Autodesk Inventor part; units mm, degrees
ref_plane "YZ Plane" through (0, 0, 0) normal (1, 0, 0) x (0, 1, 0)
ref_plane "XZ Plane" through (0, 0, 0) normal (0, 1, 0) x (-1, 0, 0)
ref_plane "XY Plane" through (0, 0, 0) normal (0, 0, 1) x (1, 0, 0)
sketch "Boceto2" plane through (0, 0, 0) normal (0, 0, 1) x (1, 0, 0)
  circle A0 centre (0, 0) radius 7.9375
  dimension "d0" = 15.875
extrude "Extrusión1" add sketch "Boceto2" against normal blind 815
sketch "Boceto3" plane through (0, 0, 0) normal (0, 0, 1) x (1, 0, 0)
  circle A0 centre (0, 0) radius 7.9375
extrude "Extrusión2" add sketch "Boceto3" along normal blind 4
sketch "Boceto6" plane through (0, 0, 4) normal (0, 0, 1) x (1, 0, 0)
  circle A0 centre (0, 0) radius 3
  dimension "d15" = 6
sketch "Boceto7" plane through (0, 0, -815) normal (0, 0, -1) x (-1, 0, 0)
  circle A0 centre (0, 0) radius 3
  dimension "d16" = 6
hole "Agujero1" at (0, 0, -815) direction (0, 0, 1) diameter 6 depth 10 tip angle 118
hole "Agujero2" at (0, 0, 4) direction (0, 0, -1) diameter 6 depth 10 tip angle 118
thread "Rosca3"
thread "Rosca5"
properties part number "barra" material "Acero inoxidable AISI 304"
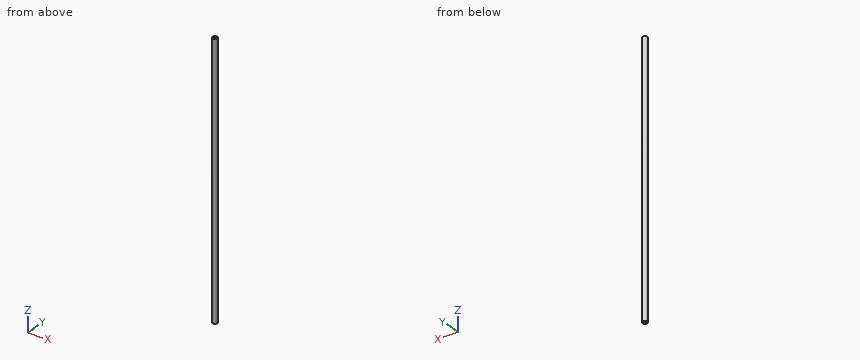
Geometry check sheet. Reference: the model listing, model coordinates, mm. Give positions to 0.01 mm unless a question says otherwise; leave off trailing zeros. Write each loop counter-clockwise with the first axis right and the second up, starting at its lowest first coordinate (ties: lowest second). Pieces come first, ordered by that corner, then holes.
1) Cross-section at A-A (z = -123.5). Record the boundary of the cut face in (x, y) (1 decimal).
Values follow:
outline: circle Ø15.9 at (0, 0)
2) Go/stop test with flat-tipped pins: pin 1 Ø1 at (y, z) = (2.5, -234) entering from +X; pin 2 Ø4 at (y, z) = (1, -728.5) entering from -X; pin 3 Ø5 at (x, y) = (0, 0) entering from +Z; pin 4 Ø5.5 at (x, y) = (0, 0) entering from -Z. Record where each tip stops, or that it passes through.
Values follow:
pin 1: stops at x = 7.68
pin 2: stops at x = -7.94
pin 3: stops at z = -6.3
pin 4: stops at z = -804.85
3) Thickness scan on line 1 (Y direction, x = 0, z = -812.5); line 2 (X direction, y = 1.5, z = -673); line 3 (X direction, y = -2.75, z = -740.5). Record the ranges inside material, lowest first.
Values follow:
line 1: y = -7.94 to -3, 3 to 7.94
line 2: x = -7.79 to 7.79
line 3: x = -7.45 to 7.45
